For this review, take the finished solid that the model builds, in its own axes (mm). Round coordinates to 2 decimals unless told otherwise and drop trailing zeros. Order: outer loops, then holes, each group sorted by start corner. A loop starts at its lowest first (then second) coordinate and runs counter-clockwise, first axis right, second up. Notation, with made-up numbers: M 60,79 L 82,79 A30 cw 82,106 Z; hole C 49.5,-12.5 d8. An arc over 180 degrees is marked long. Use a Markdown table: item, result.
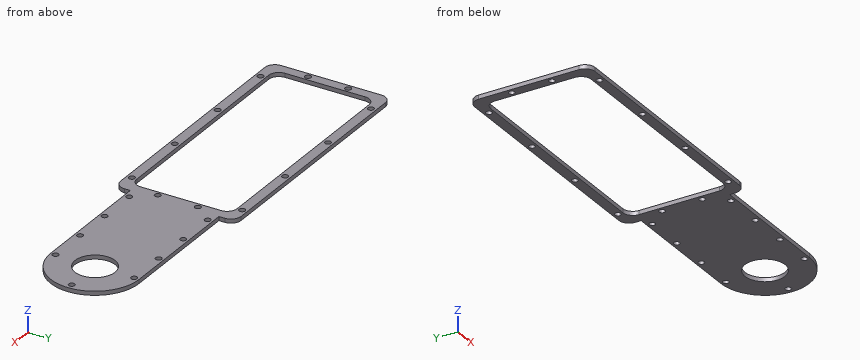
from build123d import *

# Parameters (mm, degrees)
SKETCH1_R           = 10
BOSS_EXTRUDE1_DEPTH = 2
CUT_EXTRUDE1_DEPTH  = 5
FILLET1_R           = 5
SKETCH3_R           = 1.5
CUT_EXTRUDE2_DEPTH  = 5
SKETCH4_R           = 1.5
CUT_EXTRUDE3_DEPTH  = 154.844633691


with BuildPart() as part:
    # Sketch1 → Boss-Extrude1 (new body)
    # profile 1 of 2: a face of its own
    with BuildSketch(Plane.XY):
        with BuildLine():
            Line((128.81, 22), (63.8, 22))
            Line((63.8, 22), (63.8, -22.13600286))
            Line((63.8, -22.13600286), (128.81, -22.13600286))
            ThreePointArc((128.81, -22.13600286), (150.87800143, -0.06800143), (128.81, 22))
        make_face()
        with Locations((128.81, 0)):
            Circle(SKETCH1_R, mode=Mode.SUBTRACT)
    # profile 2 of 2: a face of its own
    with BuildSketch(Plane.XY):
        with BuildLine():
            Line((-58.8, 30), (58.8, 30))
            ThreePointArc((58.8, 30), (62.335533906, 28.535533906), (63.8, 25))
            Line((63.8, 25), (63.8, -25))
            ThreePointArc((63.8, -25), (62.335533906, -28.535533906), (58.8, -30))
            Line((58.8, -30), (-58.8, -30))
            ThreePointArc((-58.8, -30), (-62.335533906, -28.535533906), (-63.8, -25))
            Line((-63.8, -25), (-63.8, 25))
            ThreePointArc((-63.8, 25), (-62.335533906, 28.535533906), (-58.8, 30))
        make_face()
    extrude(amount=BOSS_EXTRUDE1_DEPTH)

    # Sketch2 → Cut-Extrude1 (cut)
    with BuildSketch(Plane.XY.offset(2)):
        Polygon((58.8, 17), (58.8, -17.13600286), (58.8, -25), (-58.8, -25), (-58.8, 25), (58.8, 25), align=None)
    extrude(amount=-CUT_EXTRUDE1_DEPTH, mode=Mode.SUBTRACT)

    # Fillet1
    fillet1_edges = [part.edges().sort_by_distance(p)[0] for p in [
        (58.8, -25, 1),
        (-58.8, -25, 1),
        (-58.8, 25, 1),
        (58.8, 25, 1),
    ]]
    fillet(fillet1_edges, radius=FILLET1_R)

    # Sketch3 → Cut-Extrude2 (cut)
    with BuildSketch(Plane.XY.offset(2)):
        with Locations((-51.2, 27.5)):
            Circle(SKETCH3_R)
        with Locations((-16.2, 27.5)):
            Circle(SKETCH3_R)
        with Locations((18.8, 27.5)):
            Circle(SKETCH3_R)
        with Locations((53.8, 27.5)):
            Circle(SKETCH3_R)
        with Locations((61.3, 10)):
            Circle(SKETCH3_R)
        with Locations((61.3, -10)):
            Circle(SKETCH3_R)
        with Locations((53.8, -27.5)):
            Circle(SKETCH3_R)
        with Locations((18.8, -27.5)):
            Circle(SKETCH3_R)
        with Locations((-16.2, -27.5)):
            Circle(SKETCH3_R)
        with Locations((-51.2, -27.5)):
            Circle(SKETCH3_R)
        with Locations((-61.3, -10)):
            Circle(SKETCH3_R)
        with Locations((-61.3, 10)):
            Circle(SKETCH3_R)
    extrude(amount=-CUT_EXTRUDE2_DEPTH, mode=Mode.SUBTRACT)

    # Sketch4 → Cut-Extrude3 (cut, through all)
    with BuildSketch(Plane.XY.offset(2)):
        with Locations((68.81, 19.5)):
            Circle(SKETCH4_R)
        with Locations((88.81, 19.5)):
            Circle(SKETCH4_R)
        with Locations((108.81, 19.5)):
            Circle(SKETCH4_R)
        with Locations((128.81, 19.5)):
            Circle(SKETCH4_R)
        with Locations((88.81, -19.66)):
            Circle(SKETCH4_R)
        with Locations((108.81, -19.66)):
            Circle(SKETCH4_R)
        with Locations((128.81, -19.66)):
            Circle(SKETCH4_R)
        with Locations((68.81, -19.66)):
            Circle(SKETCH4_R)
        with Locations((147.81, 0)):
            Circle(SKETCH4_R)
    extrude(amount=-CUT_EXTRUDE3_DEPTH, mode=Mode.SUBTRACT)


solid = part.part
Q1. Add section A-A (x = 0). Write out the cut boundary in (y, z), then the cut area to 3 significant figures.
Determined:
| item | result |
|---|---|
| outline | M -30,0 L -25,0 L -25,2 L -30,2 Z; M 25,0 L 30,0 L 30,2 L 25,2 Z |
| area | 20.0 mm^2 |
Q2. Add section C-C (y = 4.5). Write out the cut boundary in (x, z).
Determined:
| item | result |
|---|---|
| outline | M -63.8,0 L -58.8,0 L -58.8,2 L -63.8,2 Z; M 58.8,0 L 119.88,0 L 119.88,2 L 58.8,2 Z; M 137.74,0 L 150.4,0 L 150.4,2 L 137.74,2 Z |
Q3. Wall thickness on line 1 along Y through (x, z) = (88.81, 0.8); line 2 along Y through (x, z) = (-38, 1.55); line 3 along X through (y, z) = (-5.5, 0.7): over which ranges is each line inside the solid? List them lowest first. Write a range as [from, to].
Determined:
| item | result |
|---|---|
| line 1 | y = [-22.14, -21.16], [-18.16, 18], [21, 22] |
| line 2 | y = [-30, -25], [25, 30] |
| line 3 | x = [-63.8, -58.8], [58.8, 120.46], [137.16, 150.2] |
Q4. Add section B-B (y = -15.5). Write out the cut boundary in (x, z), then the cut area to 3 significant figures.
Determined:
| item | result |
|---|---|
| outline | M -63.8,0 L -58.8,0 L -58.8,2 L -63.8,2 Z; M 58.8,0 L 144.58,0 L 144.58,2 L 58.8,2 Z |
| area | 182 mm^2 |
Q5. Clearance check with flat-ended pins moving along their axes: pin 1 (4 mm diameter, centred on x = 61.3, y = -10, fed in from -Z); pin 2 (1 mm diameter, centred on x = 91, z = 1, fed in from -Y); pin 3 (1 mm diameter, centred on y = 24, z = 1, fed in from +X); pin 4 (0.6 mm diameter, centred on y = 9.5, z = 1.5, fed in from +X). State where each tip first meets the part, or that it passes through.
Determined:
| item | result |
|---|---|
| pin 1 | stops at z = 0 |
| pin 2 | stops at y = -22.14 |
| pin 3 | stops at x = 63.8 |
| pin 4 | stops at x = 148.84 |
Q6. Add section D-D (z = 1.2). Give the number of separate pieces and of enclosed holes in the cut face, then the cut area to 3 significant figures.
Determined:
| item | result |
|---|---|
| separate pieces | 1 |
| enclosed holes | 23 |
| area | 4,950 mm^2 |
